```python
from build123d import *

# Parameters (mm, degrees)
F1_DEPTH = 63.5
F2_DEPTH = 25.4
F3_DEPTH = 7.9375
F5_R     = 6.35


with BuildPart() as f1:
    # F0 (on Front) → F1 (new body, symmetric)
    with BuildSketch(Plane.XZ):
        Polygon((-66.675, 25.4), (-66.675, -25.4), (66.675, -25.4), (66.675, 25.4), (47.625, 25.4), align=None)
    extrude(amount=F1_DEPTH, both=True)

    # F0 (on Front) → F2 (join, symmetric)
    with BuildSketch(Plane.XZ):
        with BuildLine():
            Line((47.625, 25.4), (66.675, 25.4))
            Line((66.675, 25.4), (66.675, 39.48301))
            ThreePointArc((66.675, 39.48301), (70.480936, 52.85673), (80.75818, 62.222614))
            Line((80.75818, 62.222614), (80.75818, 82.468264))
            ThreePointArc((80.75818, 82.468264), (56.869637, 66.619423), (47.625, 39.48301))
            Line((47.625, 39.48301), (47.625, 25.4))
        make_face()
        with BuildLine():
            ThreePointArc((92.075, 83.93301), (86.369391, 83.565303), (80.75818, 82.468264))
            Line((80.75818, 82.468264), (80.75818, 62.222614))
            ThreePointArc((80.75818, 62.222614), (86.262339, 64.208967), (92.075, 64.88301))
            Line((92.075, 64.88301), (117.475, 64.88301))
            Line((117.475, 64.88301), (117.475, 83.93301))
            Line((117.475, 83.93301), (92.075, 83.93301))
        make_face()
    extrude(amount=F2_DEPTH, both=True)

    # F0 (on Front) → F3 (join, symmetric)
    with BuildSketch(Plane.XZ):
        with BuildLine():
            add(Edge.make_bspline(
                [(-66.675, 25.4), (-39.794628, 53.528536), (16.976637, 85.362046), (80.75818, 84.44223)],
                knots=[0, 0, 0, 0, 159.802658, 159.802658, 159.802658, 159.802658], degree=3))
            Line((-66.675, 25.4), (47.625, 25.4))
            Line((47.625, 25.4), (47.625, 39.48301))
            ThreePointArc((47.625, 39.48301), (56.869637, 66.619423), (80.75818, 82.468264))
            Line((80.75818, 82.468264), (80.75818, 84.44223))
        make_face()
    extrude(amount=F3_DEPTH, both=True)

    # F0 (on Front) → F4 (revolve)
    with BuildSketch(Plane.XZ):
        Polygon((131.55818, 87.768322), (117.475, 87.768322), (117.475, 83.93301), (117.475, 64.88301), (117.475, 36.968322), (131.55818, 36.968322), align=None)
    revolve(axis=Axis((117.475, 0, 62.368322), (0, 0, 1)))

    # F5
    f5_edges = [f1.edges().sort_by_distance(p)[0] for p in [
        (-66.675, -63.5, 0),
        (66.675, -63.5, 0),
        (66.675, 63.5, 0),
        (-66.675, 63.5, 0),
    ]]
    fillet(f5_edges, radius=F5_R)


solid = f1.part
```
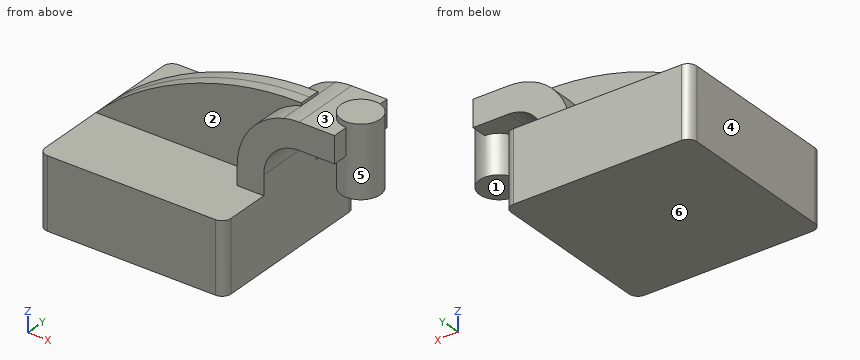
Input: part model. Units: mm. Frame: model coordinates. Face numbers are marked on the shaded views. A direction names the side the tool comes from. Round coordinates to 2 decimals unless told otherwise and drop trailing zeros. Loops run counter-clockwise (first coordinate to the right, second up) from the corner with the lowest first, then second, coordinate; pieces in that order, holes last.
1) Material intervals for line 1 (X direction, y = -22, z = 13.5) (3 decimals); line 2 (Z direction, x = 7.5, y = 40); line 3 (Z direction, x = 119, y = -2.5), sorted ascending.
Ans:
line 1: x = -66.675 to 66.675
line 2: z = -25.4 to 25.4
line 3: z = 36.97 to 87.77
2) Set-up query: the marked faces 1, 2 and 3. Return all of +Z, -Z, +X, -X, +Y, -Y with unobstructed straight access to the full face (end or side cutting, diameter ignored); none if empty.
Ans:
face 1: -Z, +X, +Y, -Y
face 2: +Z, -X, -Y
face 3: +Z
3) Pull-direction query (X, two-part tool) for the marked faces 4, 5 and 6; classes: released by +X, released by -X, zero draft, split by the parting line, or undercut.
Ans:
face 4: released by -X
face 5: undercut
face 6: zero draft
4) Section query B-B on y = 46. Return the cut outline in (x, z) (3 decimals).
Ans:
outline: (-66.675, -25.4) - (66.675, -25.4) - (66.675, 25.4) - (-66.675, 25.4) - close
5) Pin query (flat end, axial travel): pin 1 (1.6 mm diameter, centred on y = 1.5, z = 83.5, fed in from +X); pin 2 (5.5 mm diameter, centred on y = -18.5, z = 79, fed in from +X) (3 decimals); pin 3 (3 mm diameter, centred on y = -11, z = 32.5, fed in from +X) (3 decimals). Return the tip coordinate at first contact, or that it passes through.
Ans:
pin 1: stops at x = 131.54
pin 2: stops at x = 117.475
pin 3: stops at x = 66.675
6) Section query A-A on z = 22.5. Return the cut outline in (x, y) (3 decimals), plus the area to 3 significant figures.
Ans:
outline: (-66.675, -57.15) arc R6.35 ccw to (-60.325, -63.5) - (60.325, -63.5) arc R6.35 ccw to (66.675, -57.15) - (66.675, 57.15) arc R6.35 ccw to (60.325, 63.5) - (-60.325, 63.5) arc R6.35 ccw to (-66.675, 57.15) - close
area: 16,900 mm2
